Build history of the part. All positions in model axes, mm. Coordinates: 2 decimals unless noted, no trailing zeros. Order: outer loops, then holes, each group sorted by start corner. A loop starts at its lowest first (then second) coordinate and runs counter-clockwise, first axis right, second up. Notation, with made-up numbers: (28, 76) - (72, 76) arc R12 cw to (72, 82) - close; hole circle Ø8 at (-9.5, 26.5). An arc over 180 degrees is marked (long way). Return JSON: item names as keys, results as strings.
from build123d import *

# Parameters (mm, degrees)
CROQUIS1_R                    = 4
SALIENTE_EXTRUIR1_DEPTH       = 450
TALADRO_ROSCADO_M6X1_01_D     = 5
TALADRO_ROSCADO_M6X1_01_DEPTH = 17
TALADRO_ROSCADO_M6X1_01_TIP   = 1.502151548
TALADRO_ROSCADO_M6X1_02_D     = 5
TALADRO_ROSCADO_M6X1_02_DEPTH = 17
TALADRO_ROSCADO_M6X1_02_TIP   = 1.502151548


with BuildPart() as part:
    # Croquis1 → Saliente-Extruir1 (new body)
    with BuildSketch(Plane.XY):
        Circle(CROQUIS1_R)
    extrude(amount=SALIENTE_EXTRUIR1_DEPTH)

    # Taladro roscado M6x1.01
    with Locations(Plane.XY.offset(450)):
        with Locations((0, 0)):
            Hole(TALADRO_ROSCADO_M6X1_01_D / 2, depth=TALADRO_ROSCADO_M6X1_01_DEPTH)
            with Locations((0, 0, -(TALADRO_ROSCADO_M6X1_01_DEPTH + TALADRO_ROSCADO_M6X1_01_TIP / 2))):  # 118° drill point
                Cone(0, TALADRO_ROSCADO_M6X1_01_D / 2, TALADRO_ROSCADO_M6X1_01_TIP, mode=Mode.SUBTRACT)

    # Taladro roscado M6x1.02
    with Locations(Plane(origin=(0, 0, 0), x_dir=(-1, 0, 0), z_dir=(0, 0, -1))):
        with Locations((0, 0)):
            Hole(TALADRO_ROSCADO_M6X1_02_D / 2, depth=TALADRO_ROSCADO_M6X1_02_DEPTH)
            with Locations((0, 0, -(TALADRO_ROSCADO_M6X1_02_DEPTH + TALADRO_ROSCADO_M6X1_02_TIP / 2))):  # 118° drill point
                Cone(0, TALADRO_ROSCADO_M6X1_02_D / 2, TALADRO_ROSCADO_M6X1_02_TIP, mode=Mode.SUBTRACT)


solid = part.part
1. Cut at A-A on z = 289.5. Give the cut face in (x, y), plus the area to 3 significant figures.
Check values:
{"outline": "circle Ø8 at (0, 0)", "area": "50.3 mm²"}
2. Drop flat-ended pins along their axis: pin 1 (4 mm diameter, centred on x = 0, y = 0, fed in from +Z); pin 2 (2 mm diameter, centred on y = 3, z = 209.5, fed in from +X); pin 3 (2 mm diameter, centred on x = -2, z = 214.5, fed in from -Y). Give the stop position or say it passes through.
Check values:
{"pin 1": "z = 432.7", "pin 2": "x = 3.46", "pin 3": "y = -3.87"}
3. Probe L1, parallel to Y at x = 0, z = 443; L2, parallel to X at y = -0.5, z = 330.5; L3, parallel to Z at x = 1.75, y = 1.75. List the from-to ranges inside material, lowest first.
Check values:
{"L1": "-4 to -2.5, 2.5 to 4", "L2": "-3.97 to 3.97", "L3": "17.02 to 432.98"}
